Check sheet for the modelled part. Datum: model origin and axes. Units: mm. A direction names the side the tool comes from. Give positions to 0.01 mm unless a question says otherwise; leave off trailing zeros. Write each loop counter-clockwise with the first axis right and the second up, starting at its lowest first coordinate (ties: lowest second). Pieces come first, ordered by that corner, then holes. Notation, with made-up numbers: M -25.5,34 L 27.5,34 A12 cw 27.5,40 Z; hole C 79,-17.75 d6. An arc over 180 degrees is marked long. Use CSV: the item, a comma, the result in double quotes. Start each with the question number.
1. Depth check by flat-ended pin: P1, Ø5, axis at x = -10.39, y = -6, coming from the -Z side; P2, Ø1.5, axis at y = 12.5, z = 4, coming from the -X side; P3, Ø2, axis at y = 5.5, z = 2, coming from the -X side. Enter the tip coordinate at first touch or a pass-through.
2. Cross-section at D-D, the plane y = -6. State how many separate pieces and enclosed holes the cut face has, and give its area (3 significant figures).
3. Cross-section at A-A, the plane x = -4. Enter the section's corners in (y, z), and give its area (3 significant figures).
4. Access from +Z, -Z, +X, -X, +Y, -Y to the whole of each face (thin tool, end or side, straight path). Record for faces 4 (the face through (7, -7, 0)), 5 (the face through (-11.65, -0.04, 3.45)).
5. Scan lines: line 1 (Y direction, x = 0, z = 4); line 2 (X direction, y = -6.5, z = 3.5); line 3 (X direction, y = 7.5, z = 6.25). Record each from-to range of solid material in increasing order.
6. Mould release check, pull along Y, two halves, no side actions. Record for faces 1 (the face through (8.394, -5.912, 3.451)), 2 (the face through (-2.018, 15.368, 3.451)), 3 (the face through (7, -7, 7)): +Y half, -Y half, draft (parallel to the pull), parting line (faces both ways), or undercut.
7. Cross-section at C-C, the plane x = 9. Enter the section's corners in (y, z), and give its area (3 significant figures).
8. Cross-section at B-B, the plane y = 1. Enter the section's corners in (x, z), and give its area (3 significant figures).
from build123d import *

# Parameters (mm, degrees)
SKETCH_1_R      = 15.5
SKETCH_1_R_2    = 2
EXTRUDE_1_DEPTH = 7
FILLET_1_R      = 3


with BuildPart() as part:
    # 草图1 → 凸台-拉伸1 (new body)
    with BuildSketch(Plane.XY):
        Circle(SKETCH_1_R)
        with Locations((-10.392304845, -6)):
            Circle(SKETCH_1_R_2, mode=Mode.SUBTRACT)
        with Locations((0, -12)):
            Circle(SKETCH_1_R_2, mode=Mode.SUBTRACT)
        with Locations((10.392304845, -6)):
            Circle(SKETCH_1_R_2, mode=Mode.SUBTRACT)
        with Locations((-10.392304845, 6)):
            Circle(SKETCH_1_R_2, mode=Mode.SUBTRACT)
        with BuildLine():
            ThreePointArc((2.604308084, 8.091203829), (4.681947148, 10.376164045), (6.9, 8.227241336))
            ThreePointArc((6.9, 8.227241336), (6.576995231, 7.093844482), (5.705034021, 6.300998875))
            ThreePointArc((5.705034021, 6.300998875), (7.769903126, 3.446535276), (8.5, 0))
            ThreePointArc((8.5, 0), (7.769903126, -3.446535276), (5.705034021, -6.300998875))
            ThreePointArc((5.705034021, -6.300998875), (6.576995231, -7.093844482), (6.9, -8.227241336))
            ThreePointArc((6.9, -8.227241336), (4.681947148, -10.376164045), (2.604308084, -8.091203829))
            ThreePointArc((2.604308084, -8.091203829), (-4.25, -7.361215932), (-8.309342105, -1.790204954))
            ThreePointArc((-8.309342105, -1.790204954), (-11.65, 0), (-8.309342105, 1.790204954))
            ThreePointArc((-8.309342105, 1.790204954), (-4.25, 7.361215932), (2.604308084, 8.091203829))
        make_face(mode=Mode.SUBTRACT)
        with Locations((10.392304845, 6)):
            Circle(SKETCH_1_R_2, mode=Mode.SUBTRACT)
        with Locations((0, 12)):
            Circle(SKETCH_1_R_2, mode=Mode.SUBTRACT)
    extrude(amount=EXTRUDE_1_DEPTH)

    # 圆角1
    fillet_1_edges = [part.edges().sort_by_distance(p)[0] for p in [
        (-8.309342105, 1.790204954, 3.5),
        (-8.309342105, -1.790204954, 3.5),
        (2.604308084, -8.091203829, 3.5),
        (5.705034021, -6.300998875, 3.5),
        (5.705034021, 6.300998875, 3.5),
        (2.604308084, 8.091203829, 3.5),
    ]]
    fillet(fillet_1_edges, radius=FILLET_1_R)


solid = part.part
Worked answers:
1,P1,"stops at z = 0"
1,P2,"stops at x = -10.11"
1,P3,"stops at x = -14.83"
2,separate pieces,"4"
2,enclosed holes,"0"
2,area,"55.8 mm^2"
3,outline,"M -14.97,0 L -7.5,0 L -7.5,7 L -14.97,7 Z; M 7.5,0 L 14.97,0 L 14.97,7 L 7.5,7 Z"
3,area,"105 mm^2"
4,face 4,"-Z, +X, -X, +Y, -Y"
4,face 5,"+Z, -Z"
5,line 1,"y = -15.5 to -14, -10 to -8.5, 8.5 to 10, 14 to 15.5"
5,line 2,"x = -14.07 to -12.33, -8.46 to -5.48, 6.56 to 8.46, 12.33 to 14.07"
5,line 3,"x = -13.56 to -11.72, -9.07 to -4, 6.77 to 9.07, 11.72 to 13.56"
6,face 1,"undercut"
6,face 2,"parting line"
6,face 3,"draft"
7,outline,"M -12.62,0 L -7.44,0 L -7.44,7 L -12.62,7 Z; M -4.56,0 L 4.56,0 L 4.56,7 L -4.56,7 Z; M 7.44,0 L 12.62,0 L 12.62,7 L 7.44,7 Z"
7,area,"136 mm^2"
8,outline,"M -15.47,0 L -11.4,0 L -11.4,7 L -15.47,7 Z; M 8.44,0 L 15.47,0 L 15.47,7 L 8.44,7 Z"
8,area,"77.6 mm^2"
